Here's how the part is built. I have some questions about the finished solid (model axes, mm). A direction names the side the tool comes from. Round coordinates to 2 decimals unless told otherwise and drop trailing zeros. Write each loop counter-clockwise with the first axis right and the second up, starting at its lowest first coordinate (ties: lowest second). Pieces come first, ordered by that corner, then holes. Notation, with made-up numbers: M -31.5,-15 L 14.5,-15 A31 ccw 14.5,15 Z; hole C -28,-33.75 d7. An arc over 180 degrees is marked long. Write item = value, one per line. Start each with the question number.
(1) Will these pins go through, and if not, where does the flat tip stop? pin 1 Ø1.9 at (x, y) = (4.5, -28) entering from -Z; pin 2 Ø1.1 at (y, z) = (-27, -4) entering from +X.
(2) I want a section at B-B (x = 82.5). List the corners of the cut face in (y, z) for me.
(3) I want a section at D-D (y = -7.75). List the corners of the cut face in (x, z) for me (3 decimals).
(4) If we mould it in two halves opening along X, with no side actions, what happens to faces 3 (the cylindrical face through (114.9, -26.1, -148.3)), 4 (the flat face through (1.905, -27, -4)), 5 (the flat face through (3, -29.21, -4))? For each: released by +X, released by -X, zero draft, split by the parting line, or undercut.
(5) I need wall thicknesses on line 1 along Z through (x, y) = (6.35, -18.25); line 2 along Z through (x, y) = (19.5, -13); line 3 along X through (y, z) = (-11, -45) (3 decimals). Which ranges of each line are inside material? Lowest first, please.
(6) On a 3-axis mill with a long thin cutter (end or side, diameter ignored), from which of +Z, -Z, +X, -X, +Y, -Y can I reach the whole of each face in a straight line? I mean faces 1 (the flat face through (3, -29.21, -98)), 2 (the flat face through (59, -13, -139.7)). Say none if no direction works.
(7) I want a section at C-C (x = 19.05). List the corners of the cut face in (y, z) for me (3 decimals).
(8) I want a section at A-A (z = -90). List the corners of the cut face in (x, y) for me (3 decimals).
```python
from build123d import *

# Parameters (mm, degrees)
F0_W     = 120.015
F0_H     = 152.4
F0_W_2   = 3.81
F0_H_2   = 3.81
F0_R     = 3.175
F0_W_3   = 94.615
F0_H_3   = 127
F1_DEPTH = 25.4
F2_DEPTH = 29.21
F3_R     = 1.778
F4_DEPTH = 118.111
F5_DEPTH = 29.21
F6_R     = 1.778
F7_DEPTH = 150.496
F8_R     = 1.778
F9_DEPTH = 150.496


with BuildPart() as f1:
    # F0 (on Front) → F1 (new body)
    with BuildSketch(Plane.XZ):
        with Locations((60.0075, -76.2)):
            Rectangle(F0_W, F0_H)
        with Locations((3.81, -146.685)):
            Rectangle(F0_W_2, F0_H_2, mode=Mode.SUBTRACT)
        with Locations((19.05, -146.05)):
            Circle(F0_R, mode=Mode.SUBTRACT)
        with Locations((3.81, -97.79)):
            Rectangle(F0_W_2, F0_H_2, mode=Mode.SUBTRACT)
        with Locations((100.965, -146.05)):
            Circle(F0_R, mode=Mode.SUBTRACT)
        with Locations((116.205, -146.685)):
            Rectangle(F0_W_2, F0_H_2, mode=Mode.SUBTRACT)
        with Locations((116.205, -97.79)):
            Rectangle(F0_W_2, F0_H_2, mode=Mode.SUBTRACT)
        with Locations((6.35, -73.025)):
            Circle(F0_R, mode=Mode.SUBTRACT)
        with Locations((60.0075, -76.2)):
            Rectangle(F0_W_3, F0_H_3, mode=Mode.SUBTRACT)
        with Locations((6.35, -15.875)):
            Circle(F0_R, mode=Mode.SUBTRACT)
        with Locations((3.81, -3.81)):
            Rectangle(F0_W_2, F0_H_2, mode=Mode.SUBTRACT)
        with Locations((113.665, -73.025)):
            Circle(F0_R, mode=Mode.SUBTRACT)
        with Locations((113.665, -15.875)):
            Circle(F0_R, mode=Mode.SUBTRACT)
        with Locations((116.205, -3.81)):
            Rectangle(F0_W_2, F0_H_2, mode=Mode.SUBTRACT)
    extrude(amount=F1_DEPTH)

    # F0 (on Front) → F2 (join)
    with BuildSketch(Plane.XZ):
        with Locations((116.205, -146.685)):
            Rectangle(F0_W_2, F0_H_2)
        with Locations((3.81, -146.685)):
            Rectangle(F0_W_2, F0_H_2)
    extrude(amount=F2_DEPTH)

    # F3 (on face) → F4 (cut, through all)
    with BuildSketch(Plane(origin=(1.905, 0, 0), x_dir=(0, -1, 0), z_dir=(-1, 0, 0))):
        with Locations((27.305, -146.685)):
            Circle(F3_R)
    extrude(amount=-F4_DEPTH, mode=Mode.SUBTRACT)

    # F0 (on Front) → F5 (join)
    with BuildSketch(Plane.XZ):
        with Locations((116.205, -97.79)):
            Rectangle(F0_W_2, F0_H_2)
        with Locations((116.205, -3.81)):
            Rectangle(F0_W_2, F0_H_2)
        with Locations((3.81, -3.81)):
            Rectangle(F0_W_2, F0_H_2)
        with Locations((3.81, -97.79)):
            Rectangle(F0_W_2, F0_H_2)
    extrude(amount=F5_DEPTH)

    # F6 (on face) → F7 (cut, through all)
    with BuildSketch(Plane.XY.offset(-1.905)):
        with Locations((3.81, -27.305)):
            Circle(F6_R)
    extrude(amount=-F7_DEPTH, mode=Mode.SUBTRACT)

    # F8 (on face) → F9 (cut, through all)
    with BuildSketch(Plane.XY.offset(-1.905)):
        with Locations((116.205, -27.305)):
            Circle(F8_R)
    extrude(amount=-F9_DEPTH, mode=Mode.SUBTRACT)


solid = f1.part
```
Returned:
q1.pin_1 = -148.59
q1.pin_2 = 118.11
q2.outline = M -25.4,-152.4 L 0,-152.4 L 0,-139.7 L -25.4,-139.7 Z; M -25.4,-12.7 L 0,-12.7 L 0,0 L -25.4,0 Z
q3.outline = M 0,-152.4 L 120.015,-152.4 L 120.015,0 L 0,0 Z; hole C 6.35,-73.025 d6.35; hole C 6.35,-15.875 d6.35; hole M 12.7,-139.7 L 107.315,-139.7 L 107.315,-12.7 L 12.7,-12.7 Z; hole C 19.05,-146.05 d6.35; hole C 100.965,-146.05 d6.35; hole C 113.665,-73.025 d6.35; hole C 113.665,-15.875 d6.35
q4.face_3 = undercut
q4.face_4 = released by -X
q4.face_5 = zero draft
q5.line_1 = -152.4 to -76.2, -69.85 to -19.05, -12.7 to 0
q5.line_2 = -152.4 to -149.19, -142.91 to -139.7, -12.7 to 0
q5.line_3 = 0 to 12.7, 107.315 to 120.015
q6.face_1 = +Z, -Z, +X, -X, -Y
q6.face_2 = +Y, -Y
q7.outline = M -25.4,-152.4 L 0,-152.4 L 0,-149.225 L -25.4,-149.225 Z; M -25.4,-142.875 L 0,-142.875 L 0,-139.7 L -25.4,-139.7 Z; M -25.4,-12.7 L 0,-12.7 L 0,0 L -25.4,0 Z
q8.outline = M 0,-25.4 L 12.7,-25.4 L 12.7,0 L 0,0 Z; M 107.315,-25.4 L 120.015,-25.4 L 120.015,0 L 107.315,0 Z
